Could you check a few things on this model? Use its own coordinates, in mm. A direction names the side the tool comes from. Give positions to 0.01 mm unless a question says otherwise; leave off trailing zeros. Order: outer loops, then holes, each group sorted by start corner. A loop starts at its lowest first (then second) coordinate and runs counter-clockwise, first axis right, second up.
(1) Imagine slicing it at A-A, the plane y = 45.5. Write out the boundary of the cut face in (x, z), then the cut area to 3 significant figures.
(2) Imagine slicing it at D-D, the plane z = -24. Write out the boundary of the cut face in (x, y), then the cut area to 3 significant figures.
(3) If we mould it in two halves opening along X, with no side actions, what happens to faces 1 (the flat face through (6, 20, -36)), 2 (the flat face through (14, 0, -28)), 3 (the flat face through (14, 38.3, -54))? For each: released by +X, released by -X, zero draft, split by the parting line, or undercut.
(4) Imagine slicing it at C-C, the plane x = 15.5. Write out the boundary of the cut face in (y, z).
(5) Will these pins go through, and if not, where does the flat tip stop? pin 1 (1 mm diameter, centred on x = 16.5, z = -44.5, fed in from +Y); pin 2 (3 mm diameter, centred on x = 15.5, y = 8, fed in from +Z).
(6) If I drill on probe 1 along Z at (x, y) = (24.75, 39.5); probe 2 along Y at (x, z) = (26.5, -4.5), over which ranges is the centre line in solid material (lowest first)?
(7) Imagine slicing it at B-B, the plane z = -18. Write out the boundary of the cut face in (x, y), then the cut area to 3 significant figures.
(8) On a 3-axis mill with a long thin cutter (end or side, diameter ignored), from which of +Z, -Z, +X, -X, +Y, -Y can I reach the whole of each face in a straight line? I mean faces 4 (the flat face through (17.2, 44, -54)), 5 (the flat face through (17.2, 3, -13)), 6 (the cylindrical face through (27.4, 2.96, -0.57)). Say none if no direction works.
from build123d import *

# Parameters (mm, degrees)
SALIENTE_EXTRUIR1_DEPTH = 28
VACIADO2_START          = 6
VACIADO2_OUTLINE_W      = 22
VACIADO2_OUTLINE_H      = 53
VACIADO2_DEPTH          = 51
CORTAR_EXTRUIR1_REACH   = 83.449
CROQUIS2_W              = 6.4
CROQUIS2_H              = 11
CROQUIS2_H_2            = 10
CORTAR_EXTRUIR2_REACH   = 83.449
CROQUIS5_W              = 6.4
CROQUIS5_H              = 10
CROQUIS5_H_2            = 11
REDONDEO2_R             = 2


# Read off the part's stored shape, not the designer's step: Vaciado2
with BuildPart() as part:
    # Croquis1 → Saliente-Extruir1 (new body)
    with BuildSketch(Plane(origin=(0, 0, 0), x_dir=(0, 0, -1), z_dir=(1, 0, 0))):
        Polygon((0, 0), (57, 0), (57, 57), (51, 57), (0, 6), align=None)
    extrude(amount=SALIENTE_EXTRUIR1_DEPTH)

    # Vaciado2 outline → Vaciado2 (cut)
    with BuildSketch(Plane(origin=(0, 0, 0), x_dir=(1, 0, 0), z_dir=(0, 1, 0)).offset(VACIADO2_START)):
        with Locations((17, 24.5)):
            Rectangle(VACIADO2_OUTLINE_W, VACIADO2_OUTLINE_H)
    extrude(amount=VACIADO2_DEPTH, mode=Mode.SUBTRACT)

    # Croquis2 → Cortar-Extruir1 (cut, up to next)
    with BuildSketch(Plane.XY.offset(-51), mode=Mode.PRIVATE) as cortar_extruir1_sk1:
        with Locations((14, 43.8)):
            Rectangle(CROQUIS2_W, CROQUIS2_H)
    cortar_extruir1_tool1 = extrude(cortar_extruir1_sk1.sketch, amount=-CORTAR_EXTRUIR1_REACH, mode=Mode.PRIVATE) & part.part
    # Croquis2 → Cortar-Extruir1 (cut, up to next)
    with BuildSketch(Plane.XY.offset(-51), mode=Mode.PRIVATE) as cortar_extruir1_sk2:
        with Locations((14, 15)):
            Rectangle(CROQUIS2_W, CROQUIS2_H_2)
    cortar_extruir1_tool2 = extrude(cortar_extruir1_sk2.sketch, amount=-CORTAR_EXTRUIR1_REACH, mode=Mode.PRIVATE) & part.part
    add(cortar_extruir1_tool1.solids().sort_by_distance((14, 43.8, -51))[0], mode=Mode.SUBTRACT)
    add(cortar_extruir1_tool2.solids().sort_by_distance((14, 15, -51))[0], mode=Mode.SUBTRACT)

    # Croquis5 → Cortar-Extruir2 (cut, up to next)
    with BuildSketch(Plane(origin=(0, 6, 0), x_dir=(1, 0, 0), z_dir=(0, 1, 0)), mode=Mode.PRIVATE) as cortar_extruir2_sk1:
        with Locations((14, 42)):
            Rectangle(CROQUIS5_W, CROQUIS5_H)
    cortar_extruir2_tool1 = extrude(cortar_extruir2_sk1.sketch, amount=-CORTAR_EXTRUIR2_REACH, mode=Mode.PRIVATE) & part.part
    # Croquis5 → Cortar-Extruir2 (cut, up to next)
    with BuildSketch(Plane(origin=(0, 6, 0), x_dir=(1, 0, 0), z_dir=(0, 1, 0)), mode=Mode.PRIVATE) as cortar_extruir2_sk2:
        with Locations((14, 13.2)):
            Rectangle(CROQUIS5_W, CROQUIS5_H_2)
    cortar_extruir2_tool2 = extrude(cortar_extruir2_sk2.sketch, amount=-CORTAR_EXTRUIR2_REACH, mode=Mode.PRIVATE) & part.part
    add(cortar_extruir2_tool1.solids().sort_by_distance((14, 6, -42))[0], mode=Mode.SUBTRACT)
    add(cortar_extruir2_tool2.solids().sort_by_distance((14, 6, -13.2))[0], mode=Mode.SUBTRACT)

    # Redondeo2
    redondeo2_edges = [part.edges().sort_by_distance(p)[0] for p in [
        (28, 3, 0),
        (28, 57, -54),
        (0, 3, 0),
        (0, 57, -54),
    ]]
    fillet(redondeo2_edges, radius=REDONDEO2_R)


solid = part.part
Answer block:
1. outline: (0, -57) - (10.8, -57) - (10.8, -51) - (6, -51) - (6, -39.5) - (0, -39.5) - close; (17.2, -57) - (28, -57) - (28, -51) - (17.2, -51) - close
1. area: 199 mm2
2. outline: (0, 0) - (28, 0) - (28, 6) - (6, 6) - (6, 30) - (0, 30) - close
2. area: 312 mm2
3. face 1: released by +X
3. face 2: zero draft
3. face 3: undercut
4. outline: (0, -57) - (10, -57) - (10, -51) - (6, -51) - (6, -47) - (0, -47) - close; (0, -37) - (6, -37) - (6, -18.7) - (0, -18.7) - close; (0, -7.7) - (6, -7.7) - (6, 0) - (0, 0) - close; (20, -57) - (38.3, -57) - (38.3, -51) - (20, -51) - close; (49.3, -57) - (57, -57) - (57, -51) - (49.3, -51) - close
5. pin 1: passes through
5. pin 2: stops at z = -51
6. probe 1: z = -57 to -51
6. probe 2: y = 0 to 6
7. outline: (0, 0) - (10.8, 0) - (10.8, 6) - (6, 6) - (6, 24) - (0, 24) - close; (17.2, 0) - (28, 0) - (28, 6) - (17.2, 6) - close
7. area: 238 mm2
8. face 4: +Z, -Z
8. face 5: +Y, -Y
8. face 6: +Z, +X, +Y, -Y
